Verification items for the finished model (mm, model axes). A direction names the side the tool comes from. Give positions to 0.01 mm unless a question says otherwise; leave off trailing zeros. Write each loop counter-clockwise with the first axis right and the second up, starting at its lowest first coordinate (ties: lowest second). Pieces come first, ordered by that corner, then holes. Notation, with made-up numbers: (-30, -23) -> (16, -23) arc R27 ccw to (16, 12) -> close; hole circle Ø10 at (25.5, 56). An arc over 180 degrees is marked (long way). Use one line per item in the form item = value. Start each with the question number.
(1) Section check D-D, the plane y = 22. Record the cut outline in (x, z).
(2) Section check C-C, the plane x = 4.5. Record the cut outline in (y, z), plus the area to 3 significant figures.
(3) Set-up check for faces 5 (the face through (0, 17, 22)), 6 (the face through (0, 1, -13)): record each of +Z, -Z, +X, -X, +Y, -Y from which the full face is reachable in a straight line by a thin tool's end or side.
(4) Scan lines: L1, parallel to Y at x = 0, z = 22.85; L2, parallel to Z at x = 3.75, y = 12; L3, parallel to Y at x = -7, z = 19. Record each from-to range of solid material in increasing order.
(5) Depth check by flat-ended pin: pin 1 Ø4 at (x, y) = (9, 12.5) entering from -Z; pin 2 Ø8 at (x, z) = (-6, 6) entering from +Y. Enter the tip coordinate at first touch or a pass-through.
(6) Section check A-A, the plane x = 0. Record the cut outline in (y, z), plus the area to 3 significant figures.
(7) Section check B-B, the plane z = 9. Record the cut outline in (x, y), plus the area to 3 significant figures.
(8) Release check for a two-part mould opening along Y. For faces 1 (the face through (0, 15, 25)), 2 (the face through (0.379, 23.714, 23.479)), 3 (the face through (0, 30, 24)), 4 (the face through (0.228, 12.157, 23.479)) record: pulls with the +Y half, pulls with the -Y half, needs draft (parallel to the pull), parting line crosses it, or undercut.
from build123d import *

# Parameters (mm, degrees)
SKETCH_1_R          = 13
SKETCH_1_R_2        = 9.5
EXTRUDE_1_DEPTH     = 3
SKETCH_2_W          = 26
SKETCH_2_H          = 30
EXTRUDE_2_DEPTH     = 3
SKETCH_3_R          = 1.75
CUT_EXTRUDE_1_DEPTH = 3


with BuildPart() as part:
    # 草图1 → 凸台-拉伸1 (new body)
    # profile 1 of 2: a face of its own
    with BuildSketch(Plane(origin=(0, 0, 0), x_dir=(1, 0, 0), z_dir=(0, 1, 0))):
        Circle(SKETCH_1_R)
        with Locations(Location((0, 0, 0), (0, 0, 270))):
            Circle(SKETCH_1_R_2, mode=Mode.SUBTRACT)
    # profile 2 of 2: a face of its own
    with BuildSketch(Plane(origin=(0, 0, 0), x_dir=(1, 0, 0), z_dir=(0, 1, 0))):
        with BuildLine():
            ThreePointArc((13, 0), (0, -13), (-13, 0))
            Line((-13, 0), (-13, -25))
            Line((-13, -25), (13, -25))
            Line((13, -25), (13, 0))
        make_face()
    extrude(amount=EXTRUDE_1_DEPTH)

    # 草图2 → 凸台-拉伸2 (add)
    with BuildSketch(Plane.XY.offset(25)):
        with Locations((0, 15)):
            Rectangle(SKETCH_2_W, SKETCH_2_H)
    extrude(amount=-EXTRUDE_2_DEPTH)

    # 草图3 → 切除-拉伸1 (cut)
    with BuildSketch(Plane(origin=(0, 0, 22), x_dir=(-1, 0, 0), z_dir=(0, 0, -1))):
        with Locations((0, 10.422083653)):
            Circle(SKETCH_3_R)
        with Locations((0, 25.422083653)):
            Circle(SKETCH_3_R)
    extrude(amount=-CUT_EXTRUDE_1_DEPTH, mode=Mode.SUBTRACT)


solid = part.part
Completed:
q1.outline = (-13, 22) -> (13, 22) -> (13, 25) -> (-13, 25) -> close
q2.outline = (0, -12.2) -> (3, -12.2) -> (3, -8.37) -> (0, -8.37) -> close; (0, 8.37) -> (3, 8.37) -> (3, 22) -> (30, 22) -> (30, 25) -> (0, 25) -> close
q2.area = 142 mm²
q3.face_5 = -Z, +X, -X, +Y
q3.face_6 = -Z, +Y, -Y
q4.L1 = 0 to 8.67, 12.17 to 23.67, 27.17 to 30
q4.L2 = 22 to 25
q4.L3 = 0 to 3
q5.pin_1 = 22
q5.pin_2 = 3
q6.outline = (0, -13) -> (3, -13) -> (3, -9.5) -> (0, -9.5) -> close; (0, 9.5) -> (3, 9.5) -> (3, 22) -> (8.67, 22) -> (8.67, 25) -> (0, 25) -> close; (12.17, 22) -> (23.67, 22) -> (23.67, 25) -> (12.17, 25) -> close; (27.17, 22) -> (30, 22) -> (30, 25) -> (27.17, 25) -> close
q6.area = 117 mm²
q7.outline = (-13, 0) -> (-3.04, 0) -> (-3.04, 3) -> (-13, 3) -> close; (3.04, 0) -> (13, 0) -> (13, 3) -> (3.04, 3) -> close
q7.area = 59.8 mm²
q8.face_1 = needs draft
q8.face_2 = undercut
q8.face_3 = pulls with the +Y half
q8.face_4 = undercut
